Read the model definition and answer for the solid it produces. Units are mm, in the model's axes. Face numbers are marked on the shaded views. A direction names the side the tool comes from. Give positions to 0.01 mm unless a question says otherwise; leave off trailing zeros. Loops run counter-clockwise (first coordinate to the right, second up) from the corner with the lowest first, then second, coordinate; pieces in that order, holes last.
(1) Find section C-C, the plane x = 10.5. Write down the section's boundary in (y, z), then the cut area to 3 significant figures.
(2) Find section A-A, the plane x = 42. Write down the section's boundary in (y, z).
(3) Find section D-D, the plane z = 3.5. Write down the section's boundary in (x, y), then the cut area to 3 significant figures.
(4) Find section B-B, the plane z = 59.5. Write down the section's boundary in (x, y).
(5) Each of these flat-tipped pins is pushed along its axis until it touches: P1, Ø4.5, axis at y = 10, z = 51.2, coming from the +X side; P2, Ø6.5, axis at x = 53.5, y = 1.5, coming from the +Z side; P3, Ø2, axis at y = 2, z = 46.5, coming from the +X side; P4, Ø7, axis at x = 38.5, y = 8, coming from the +Z side. Where does it stop, or does it pass through?
(6) Straight lines are drawn through the part: probe 1 along X at (y, z) = (10, 3.75); probe 2 along Y at (x, z) = (113.25, 51.2); probe 3 along X at (y, z) = (18, 29.5). For each, find the intervals that lie inside material, in ascending order.
(7) Which of the six approach directions +Z, -Z, +X, -X, +Y, -Y give full straight-line access (tool end or side, diameter ignored) to the marked faces 1, 2 and 3?
```python
from build123d import *

# Parameters (mm, degrees)
BOSS_EXTRUDE1_DEPTH = 20
BOSS_EXTRUDE2_DEPTH = 90
SKETCH4_R           = 2.45
CUT_EXTRUDE1_DEPTH  = 137.301137193
LPATTERN1_COUNT     = 4
LPATTERN1_PITCH     = 8.3
SKETCH5_R           = 2.45
CUT_EXTRUDE2_DEPTH  = 14
LPATTERN2_COUNT     = 5
LPATTERN2_PITCH     = 9
FILLET2_R           = 5
BOSS_EXTRUDE4_DEPTH = 20
BOSS_EXTRUDE5_DEPTH = 2
LPATTERN3_COUNT     = 3
LPATTERN3_PITCH     = 9
FILLET3_R           = 0.3
FILLET4_R           = 20


with BuildPart() as part:
    # Sketch1 → Boss-Extrude1 (new body)
    with BuildSketch(Plane(origin=(0, 0, 0), x_dir=(1, 0, 0), z_dir=(0, 1, 0))):
        with BuildLine():
            Line((0, 0), (90, 0))
            ThreePointArc((90, 0), (109.091883092, -7.908116908), (117, -27))
            Line((117, -27), (117, -67))
            Line((117, -67), (110, -67))
            Line((110, -67), (110, -27))
            ThreePointArc((110, -27), (104.142135624, -12.857864376), (90, -7))
            Line((90, -7), (0, -7))
            Line((0, -7), (0, 0))
        make_face()
    extrude(amount=BOSS_EXTRUDE1_DEPTH)

    # Sketch2 → Boss-Extrude2 (add)
    with BuildSketch(Plane(origin=(0, 0, 0), x_dir=(0, 0, -1), z_dir=(1, 0, 0))):
        Polygon((-10, 15), (-10, 5), (-7, 6.398922974), (-7, 13.601077026), align=None)
    extrude(amount=BOSS_EXTRUDE2_DEPTH)

    # Sketch4 → Cut-Extrude1 (cut, through all)
    with BuildSketch(Plane(origin=(0, 0, 0), x_dir=(0, 0, -1), z_dir=(1, 0, 0))):
        with Locations(Location((-59.5, 10, 0), (0, 0, 180))):
            Circle(SKETCH4_R)
    cut_extrude1 = extrude(amount=CUT_EXTRUDE1_DEPTH, mode=Mode.SUBTRACT)

    # LPattern1: Cut-Extrude1 ×4
    with Locations(*[(0, 0, -i * LPATTERN1_PITCH) for i in range(1, LPATTERN1_COUNT)]):
        add(cut_extrude1, mode=Mode.SUBTRACT)

    # Sketch5 → Cut-Extrude2 (cut)
    with BuildSketch(Plane.XY):
        with Locations(Location((15, 10, 0), (0, 0, 90))):
            Circle(SKETCH5_R)
    cut_extrude2 = extrude(amount=CUT_EXTRUDE2_DEPTH, mode=Mode.SUBTRACT)

    # LPattern2: Cut-Extrude2 ×5
    with Locations(*[(i * LPATTERN2_PITCH, 0, 0) for i in range(1, LPATTERN2_COUNT)]):
        add(cut_extrude2, mode=Mode.SUBTRACT)

    # Fillet2
    fillet2_edges = [part.edges().sort_by_distance(p)[0] for p in [
        (0, 0, 3.5),
        (113.5, 20, 67),
        (0, 20, 3.5),
        (113.5, 0, 67),
    ]]
    fillet(fillet2_edges, radius=FILLET2_R)

    # Sketch6 → Boss-Extrude4 (add)
    with BuildSketch(Plane(origin=(0, 0, 0), x_dir=(1, 0, 0), z_dir=(0, 1, 0))):
        with BuildLine():
            Line((57.067989457, 0), (96.460545107, 3))
            ThreePointArc((96.460545107, 3), (115.383129249, -6.075834674), (117, -27))
            ThreePointArc((117, -27), (109.091883092, -7.908116908), (90, 0))
            Line((90, 0), (57.067989457, 0))
        make_face()
    extrude(amount=BOSS_EXTRUDE4_DEPTH)

    # Sketch8 → Boss-Extrude5 (add)
    with BuildSketch(Plane(origin=(0, 0, 0), x_dir=(1, 0, 0), z_dir=(0, 1, 0))):
        with BuildLine():
            ThreePointArc((90, -7), (102.578584062, -14.421415938), (110, -27))
            ThreePointArc((110, -27), (104.142135624, -12.857864376), (90, -7))
        make_face()
    boss_extrude5 = extrude(amount=BOSS_EXTRUDE5_DEPTH)

    # LPattern3: Boss-Extrude5 ×3
    with Locations(*[(0, i * LPATTERN3_PITCH, 0) for i in range(1, LPATTERN3_COUNT)]):
        add(boss_extrude5)

    # Fillet3
    fillet3_edges = [part.edges().sort_by_distance(p)[0] for p in [
        (45, 13.601077026, 7),
        (45, 15, 10),
        (45, 5, 10),
        (45, 6.398922974, 7),
    ]]
    fillet(fillet3_edges, radius=FILLET3_R)

    # Fillet4
    # the kernel refuses this fillet: 20 mm, written as the material it adds along each edge
    with BuildSketch(Plane(origin=(57.067989457, 0, 0), x_dir=(0.9971126456779296, 0, -0.07593663035162816), z_dir=(0, 1, 0))) as fillet4_piece_1:
        with BuildLine():
            CenterArc((FILLET4_R * 0.0380232084134, FILLET4_R), FILLET4_R, 265.644959248, 4.355040752)
            Line((-FILLET4_R * 0.0379134219382, FILLET4_R * 0.00288735432207), (0, 0))
            Line((0, 0), (FILLET4_R * 0.0380232084134, 0))
        make_face()
    extrude(amount=20)


solid = part.part
```
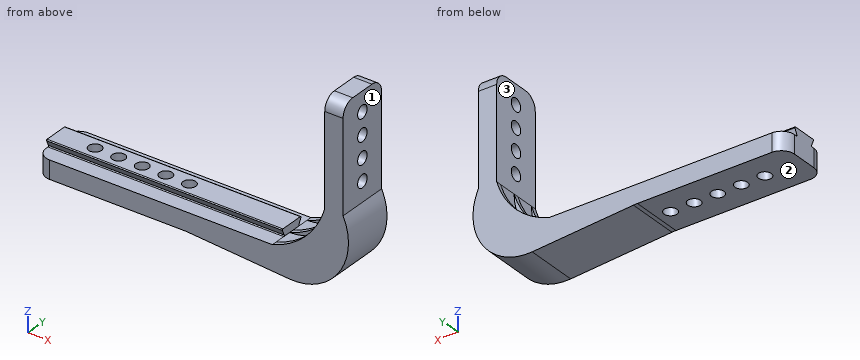
Entries:
1. outline: (0, 0) - (20, 0) - (20, 7) - (14.07, 7) arc R0.3 cw to (13.8, 7.43) - (14.8, 9.57) arc R0.3 ccw to (14.53, 10) - (5.47, 10) arc R0.3 ccw to (5.2, 9.57) - (6.2, 7.43) arc R0.3 cw to (5.93, 7) - (0, 7) - close
1. area: 166 mm2
2. outline: (0, 0) - (7.55, 0) - (7.55, 10) - (5.47, 10) arc R0.3 ccw to (5.2, 9.57) - (6.2, 7.43) arc R0.3 cw to (5.93, 7) - (0, 7) - close; (12.45, 0) - (20, 0) - (20, 7) - (14.07, 7) arc R0.3 cw to (13.8, 7.43) - (14.8, 9.57) arc R0.3 ccw to (14.53, 10) - (12.45, 10) - close
3. outline: (0, 5) arc R5 ccw to (5, 0) - (113.3, 0) - (113.3, 20) - (5, 20) arc R5 ccw to (0, 15) - close; hole circle Ø4.9 at (15, 10); hole circle Ø4.9 at (24, 10); hole circle Ø4.9 at (33, 10); hole circle Ø4.9 at (42, 10); hole circle Ø4.9 at (51, 10)
3. area: 2,160 mm2
4. outline: (110, 0) - (117, 0) - (117, 7.55) - (110, 7.55) - close; (110, 12.45) - (117, 12.45) - (117, 20) - (110, 20) - close
5. P1: passes through
5. P2: stops at z = 7
5. P3: stops at x = 117
5. P4: stops at z = 10
6. probe 1: x = 0 to 12.55, 17.45 to 21.55, 26.45 to 30.55, 35.45 to 39.55, 44.45 to 48.55, 53.45 to 113.54
6. probe 2: y = 0 to 7.55, 12.45 to 20
6. probe 3: x = 110 to 117
7. face 1: +Z, +X, +Y, -Y
7. face 2: -Z, -X, +Y, -Y
7. face 3: +Z, -X, +Y, -Y
